Input: part model. Units: mm. Frame: model coordinates. A direction names the side the tool comes from. Give positions to 0.01 mm unless a question says otherwise; leave off trailing zeros. Loops run counter-clockwise (first coordinate to the right, second up) from the corner with the lowest first, then second, coordinate; pieces in that order, holes last. Notation, with made-up numbers: M -25,-35 L -3,-35 A37 cw -3,3 Z; hole C -11,49 d7. An arc over 180 degrees is marked long. Use CSV: the item, a comma, the result in double quotes. Start each with the question number.
Q1. Section C-C, the plane y = 0.35. Output: boundary loops of the cut face in (x, z).
Q2. Reachability of faces 3 (the flat face through (265, 2.032, -33)), 4 (the cylindrical face through (267.784, 2.251, -1.162)), 5 (the cylindrical face through (286.628, -2.251, -29.807)) from +Z, -Z, +X, -X, +Y, -Y: full face, straight path, thin tool, end or side. Return the list, or none.
Q3. Pin query (flat end, axial travel): pin 1 (1 mm diameter, centred on x = 269.5, z = 43, fed in from -Y); pin 2 (2 mm diameter, centred on y = -1, z = -43.5, fed in from +X); pin 3 (9.5 mm diameter, centred on x = 273.02, z = 0, fed in from -Y); pin 4 (1.5 mm diameter, centred on x = 121, y = 0.5, fed in from -Z). Return the tip coordinate at first contact, or that it passes through.
Q4. Pull-direction query (X, two-part tool) for faces 1 (the cylindrical face through (26.55, 2.25, -1.16)), 2 (the flat face through (16, -2.464, 23)); classes: released by +X, released by -X, zero draft, split by the parting line, or undercut.
Q5. Section A-A, the plane x = 152.4. Output: boundary loops of the cut face in (y, z), plus the area to 3 significant figures.
Q6. Material intervals for line 1 along Y through (x, z) = (46.5, 64); line 2 along Z through (x, y) = (26, -0.05); line 3 along Z through (x, y) = (76.5, -1.2), sorted ascending.
Q7. Section B-B, the plane z = 0. Output: boundary loops of the cut face in (x, y), plus the area to 3 significant figures.
from build123d import *

# Parameters (mm, degrees)
SKETCH3_R          = 5.360033356
CUT_EXTRUDE1_DEPTH = 0.4318


with BuildPart() as part:
    # Sketch2 → Revolve1 (revolve)
    with BuildSketch(Plane.XY, mode=Mode.PRIVATE) as revolve1_sk:
        with BuildLine():
            Line((0, 2.4638), (38.1, 2.4638))
            Line((38.1, 2.4638), (38.1, 2.032))
            Line((38.1, 2.032), (0, 2.032))
            ThreePointArc((0, 2.032), (-2.032, 0), (0, -2.032))
            Line((0, -2.032), (14.902441519, -2.032))
            Line((14.902441519, -2.032), (14.902441519, -2.4638))
            Line((14.902441519, -2.4638), (0, -2.4638))
            ThreePointArc((0, -2.4638), (-2.4638, 0), (0, 2.4638))
        make_face()
    revolve(revolve1_sk.sketch.rotate(Axis((152.4, 15.515798555, 0), (0, -1, 0)), 270), axis=Axis((152.4, 15.515798555, 0), (0, -1, 0)))

    # Sketch3 → Cut-Extrude1 (cut)
    with BuildSketch(Plane(origin=(0, 2.4638, 0), x_dir=(1, 0, 0), z_dir=(0, 1, 0))):
        with Locations(Location((31.78326852, 0, 0), (0, 0, 270))):
            Circle(SKETCH3_R)
        with Locations(Location((152.4, 120.61673148, 0), (0, 0, 270))):
            Circle(SKETCH3_R)
        with Locations(Location((273.01673148, 0, 0), (0, 0, 270))):
            Circle(SKETCH3_R)
        with Locations(Location((152.4, -120.61673148, 0), (0, 0, 270))):
            Circle(SKETCH3_R)
    extrude(amount=-CUT_EXTRUDE1_DEPTH, mode=Mode.SUBTRACT)


solid = part.part
A:
1,outline,"C 152.4,0 d309.68; hole C 152.4,0 d308.8"
2,face 3,"none"
2,face 4,"+Y, -Y"
2,face 5,"-Y"
3,pin 1,"y = 2.03"
3,pin 2,"x = 301.23"
3,pin 3,"through"
3,pin 4,"z = -151.78"
4,face 1,"undercut"
4,face 2,"zero draft"
5,outline,"M -2.46,-152.4 A2.46 ccw 2.46,-152.4 L 2.46,-125.98 L 2.03,-125.98 L 2.03,-152.4 A2.03 cw -2.03,-152.4 L -2.03,-137.5 L -2.46,-137.5 Z; M -2.46,137.5 L -2.03,137.5 L -2.03,152.4 A2.03 cw 2.03,152.4 L 2.03,125.98 L 2.46,125.98 L 2.46,152.4 A2.46 ccw -2.46,152.4 Z; M 2.03,-115.26 L 2.46,-115.26 L 2.46,-114.3 L 2.03,-114.3 Z; M 2.03,114.3 L 2.46,114.3 L 2.46,115.26 L 2.03,115.26 Z"
5,area,"42.6 mm^2"
6,line 1,"2.03 to 2.46"
6,line 2,"-89.47 to -88.72, 88.72 to 89.47"
6,line 3,"-134.63 to -134.04, 134.04 to 134.63"
7,outline,"M 0,-2.46 L 14.9,-2.46 L 14.9,-2.03 L 0,-2.03 A2.03 cw 0,2.03 L 26.42,2.03 L 26.42,2.46 L 0,2.46 A2.46 ccw Z; M 37.14,2.03 L 38.1,2.03 L 38.1,2.46 L 37.14,2.46 Z; M 266.7,2.03 L 267.66,2.03 L 267.66,2.46 L 266.7,2.46 Z; M 278.38,2.03 L 304.8,2.03 A2.03 cw 304.8,-2.03 L 289.9,-2.03 L 289.9,-2.46 L 304.8,-2.46 A2.46 ccw 304.8,2.46 L 278.38,2.46 Z"
7,area,"42.6 mm^2"
